```python
from build123d import *

# Parameters (mm, degrees)
F0_R          = 9.525
F0_R_2        = 7.14375
F1_DEPTH      = 855.98
F1_DEPTH_BACK = 855.98
F2_R          = 7.14375
F3_DEPTH      = 906.78
F3_DEPTH_BACK = 906.78


# Not quite as in the source:
# - a feature names something its author has since deleted; it is built from what else it names


with BuildPart() as f1:
    # F0 (on Front) → F1 (new body, two sides)
    with BuildSketch(Plane.XZ) as f1_sk:
        Circle(F0_R)
        Circle(F0_R_2, mode=Mode.SUBTRACT)
    extrude(amount=F1_DEPTH)
    extrude(f1_sk.sketch, amount=-F1_DEPTH_BACK)

    # F2 (on Front) → F3 (join, two sides)
    with BuildSketch(Plane.XZ) as f3_sk:
        Circle(F2_R)
    extrude(amount=F3_DEPTH)
    extrude(f3_sk.sketch, amount=-F3_DEPTH_BACK)


solid = f1.part
```
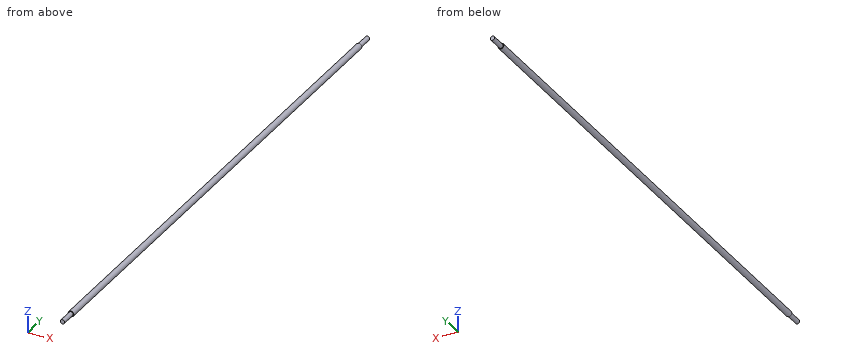
Input: part model. Units: mm. Frame: model coordinates. Round coordinates to 2 decimals unless told otherwise and drop trailing zeros. Loops run counter-clockwise (first coordinate to the right, second up) from the corner with the lowest first, then second, coordinate; pieces in that order, holes last. Notation, with made-up numbers: (64.25, -17.5) -> (89.25, -17.5) arc R18 cw to (89.25, -1.5) -> close; hole circle Ø2 at (85.25, -1.75). An arc over 180 degrees is marked (long way). One line per item, written item: value.
(1) Section C-C (x = 3.75). Return the cut outline in (y, z), plus the area to 3 significant figures.
Geometry check:
outline: (-906.78, -6.08) -> (-855.98, -6.08) -> (-855.98, -8.76) -> (855.98, -8.76) -> (855.98, -6.08) -> (906.78, -6.08) -> (906.78, 6.08) -> (855.98, 6.08) -> (855.98, 8.76) -> (-855.98, 8.76) -> (-855.98, 6.08) -> (-906.78, 6.08) -> close
area: 31,200 mm2
(2) Section A-A (y = 394). Return the cut outline in (x, z) (3 decimals).
Geometry check:
outline: circle Ø19.05 at (0, 0)
(3) Section B-B (z = 4). Return the cut outline in (x, y), plus the area to 3 significant figures.
Geometry check:
outline: (-8.64, -855.98) -> (-5.92, -855.98) -> (-5.92, -906.78) -> (5.92, -906.78) -> (5.92, -855.98) -> (8.64, -855.98) -> (8.64, 855.98) -> (5.92, 855.98) -> (5.92, 906.78) -> (-5.92, 906.78) -> (-5.92, 855.98) -> (-8.64, 855.98) -> close
area: 30,800 mm2
(4) Pin query (flat end, axial travel): pin 1 (2 mm diameter, centred on x = -7, y = -99, fed in from +Z); pin 2 (5 mm diameter, centred on x = 5.5, y = 181, fed in from +Z); pin 3 (6 mm diameter, centred on x = 7, y = -147, fed in from +Z). Return the tip coordinate at first contact, or that it passes through.
Geometry check:
pin 1: z = 7.4
pin 2: z = 9.04
pin 3: z = 8.64
(5) Material intervals for line 1 (Z direction, x = -2, y = 208.5); line 2 (Y direction, x = 7.5, z = 5.5); line 3 (Z direction, x = -1, y = -689.5), sorted ascending. Write a range as [from, to].
Geometry check:
line 1: [-9.31, 9.31]
line 2: [-855.98, 855.98]
line 3: [-9.47, 9.47]
